For this review, take the finished solid that the model builds, in its own axes (mm). Face numbers are marked on the shaded views. A direction names the side the tool comes from. Give positions to 0.01 mm unless a question says otherwise; leave off trailing zeros. Order: outer loops, then holes, each group sorted by start corner. A loop starts at its lowest first (then second) coordinate and runs counter-clockwise, first axis right, second up. Notation, with made-up numbers: (83.25, 82) -> (104.25, 82) arc R27 cw to (104.25, 102) -> close; hole circle Ø7 at (11.25, 39.5). An arc over 180 degrees is marked (long way). Return JSON: item names as keys, results as strings. Group by question number.
1) Add section D-D (x = 80). Give the boundary of the cut face in (y, z), then the cut area to 3 significant figures.
2) For the marked faces 5 and 6, list the 3-axis set-ups (+Z, -Z, +X, -X, +Y, -Y) from which the entire face can be reached by the end or side of a thin tool; tool diameter is ignored.
3) Add section C-C (z = 15.75). Give the boundary of the cut face in (x, y), then the cut area to 3 significant figures.
4) Add section A-A (y = 16). Give the boundary of the cut face in (x, z), then the cut area to 4 significant figures.
5) To check wall thickness, follow line 1 along X through (y, z) = (40.5, 10); line 2 along X through (y, z) = (-32.5, 13.5); line 3 along X through (y, z) = (34, 10.5). State the ranges of each line that lie inside material, in increasing order.
6) Insertion check: P1, Ø8.5, axis at x = 80, z = 10, coming from the +Y side. The pin has a flat end and moves straight along its axis. Give the tip position at first contact, or say it passes through.
7) The part is to be moulded in two halves that separate along X. For the marked faces 1, 2, 3 and 4, say which applies: released by +X, released by -X, zero draft, split by the parting line, or undercut.
8) Add section B-B (x = 17). Give the boundary of the cut face in (y, z), then the cut area to 3 significant figures.
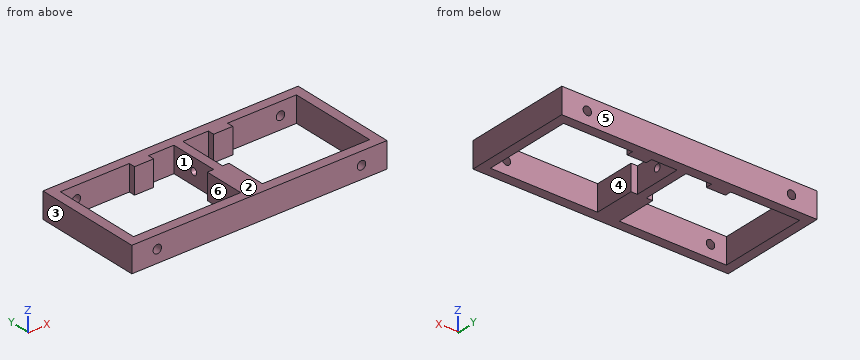
Autodesk Fusion 360 part; units mm, degrees
sketch "Sketch1" plane through (0, 0, 0) normal (0, 0, 1) x (1, 0, 0)
  line L0 (80, 0) -> (-80, 0) construction
  line L1 (100, 42.5) -> (-100, 42.5)
  line L2 (-100, 42.5) -> (-100, -42.5)
  line L3 (-100, -42.5) -> (100, -42.5)
  line L4 (100, -42.5) -> (100, 42.5)
  circle A0 centre (80, 0) radius 2.75
  circle A1 centre (-80, 0) radius 2.75
  line L5 (-90, 35) -> (-3.5, 35)
  line L6 (3.5, 35) -> (90, 35)
  line L7 (3.5, -35) -> (90, -35)
  line L8 (-3.5, -35) -> (-90, -35)
  line L9 (-3.5, 35) -> (-3.5, -3)
  line L10 (3.5, -3) -> (3.5, 35)
  line L11 (3.5, -3) -> (8.5, -3)
  line L12 (-3.5, -3) -> (-8.5, -3)
  line L13 (8.5, -3) -> (8.5, -35)
  line L14 (-8.5, -3) -> (-8.5, -35)
  line L15 (-90, 35) -> (-92.5, 35)
  line L16 (-92.5, 35) -> (-92.5, -35)
  line L17 (-92.5, -35) -> (-90, -35)
  line L18 (90, 35) -> (92.5, 35)
  line L19 (92.5, 35) -> (92.5, -35)
  line L20 (92.5, -35) -> (90, -35)
  line L21 (-23.5, 35) -> (-23.5, 30)
  line L22 (-23.5, 30) -> (-38.5, 30)
  line L23 (-38.5, 30) -> (-38.5, 35)
  line L24 (23.5, 35) -> (23.5, 30)
  line L25 (23.5, 30) -> (38.5, 30)
  line L26 (38.5, 30) -> (38.5, 35)
  dimension "d9" = 160
  dimension "d12" = 200
  dimension "d13" = 85
  dimension "d14" = 5.5
  dimension "d15" = 5.5
  dimension "d46" = 7
  dimension "d47" = 38
  dimension "d55" = 5
  dimension "d56" = 5
  dimension "d66" = 2.5
  dimension "d67" = 2.5
  dimension "d68" = 20
  dimension "d69" = 15
  dimension "d70" = 20
  dimension "d71" = 15
sketch "Sketch3" plane through (0, -42.5, 0) normal (0, -1, 0) x (1, 0, 0)
  line L0 (-100, 0) -> (100, 0)
  line L1 (100, 0) -> (100, 20)
  line L2 (100, 20) -> (-100, 20)
  line L3 (-100, 20) -> (-100, 0)
  line L4 (-100, 10) -> (-80, 10) construction
  line L5 (100, 10) -> (80, 10) construction
  dimension "d50" = 20
  dimension "d51" = 20
sketch "Sketch4" plane through (-3.5, 0, 0) normal (-1, 0, 0) x (0, -1, 0)
  line L0 (-35, 0) -> (3, 0)
  line L1 (3, 0) -> (3, 20)
  line L2 (3, 20) -> (-35, 20)
  line L3 (-35, 20) -> (-35, 0)
  line L4 (-35, 10) -> (3, 10) construction
  line L5 (-16, 20) -> (-16, 0) construction
  circle A0 centre (-16, 10) radius 2.75
  dimension "d62" = 5.5
extrude "Extrude7" add sketch "Sketch1" along normal blind 20 contours L1 L2 L3 L4 | L5 L21 L22 L23 | L6 L24 L25 L26
hole "Hole6" at (-80, -42.5, 10) at (80, -42.5, 10) direction (0, 1, 0) diameter 6.6 depth 85 tip angle 180
hole "Hole7" at (-3.5, 16, 10) direction (1, 0, 0) diameter 5.5 depth 7 tip angle 180
Evaluation:
{
 "1": {"outline": "(-42.5, 0) -> (-35, 0) -> (-35, 6.7) -> (-42.5, 6.7) -> close; (-42.5, 13.3) -> (-35, 13.3) -> (-35, 20) -> (-42.5, 20) -> close; (35, 0) -> (42.5, 0) -> (42.5, 6.7) -> (35, 6.7) -> close; (35, 13.3) -> (42.5, 13.3) -> (42.5, 20) -> (35, 20) -> close", "area": "201 mm^2"},
 "2": {"face 5": "+Z, -Z, +X, -X, +Y", "face 6": "+Z, -Z"},
 "3": {"outline": "(-100, -42.5) -> (100, -42.5) -> (100, 42.5) -> (-100, 42.5) -> close; hole (-92.5, -35) -> (-8.5, -35) -> (-8.5, -3) -> (-3.5, -3) -> (-3.5, 35) -> (-23.5, 35) -> (-23.5, 30) -> (-38.5, 30) -> (-38.5, 35) -> (-92.5, 35) -> close; hole (3.5, -3) -> (8.5, -3) -> (8.5, -35) -> (92.5, -35) -> (92.5, 35) -> (38.5, 35) -> (38.5, 30) -> (23.5, 30) -> (23.5, 35) -> (3.5, 35) -> close", "area": "5,010 mm^2"},
 "4": {"outline": "(-100, 0) -> (-92.5, 0) -> (-92.5, 20) -> (-100, 20) -> close; (-3.5, 0) -> (3.5, 0) -> (3.5, 7.25) -> (-3.5, 7.25) -> close; (-3.5, 12.75) -> (3.5, 12.75) -> (3.5, 20) -> (-3.5, 20) -> close; (92.5, 0) -> (100, 0) -> (100, 20) -> (92.5, 20) -> close", "area": "401.5 mm^2"},
 "5": {"line 1": "-100 to -83.3, -76.7 to 76.7, 83.3 to 100", "line 2": "-100 to -92.5, -8.5 to 8.5, 92.5 to 100", "line 3": "-100 to -92.5, -38.5 to -23.5, -3.5 to 3.5, 23.5 to 38.5, 92.5 to 100"},
 "6": {"P1": "y = 42.5"},
 "7": {"face 1": "undercut", "face 2": "zero draft", "face 3": "released by -X", "face 4": "undercut"},
 "8": {"outline": "(-42.5, 0) -> (-35, 0) -> (-35, 20) -> (-42.5, 20) -> close; (35, 0) -> (42.5, 0) -> (42.5, 20) -> (35, 20) -> close", "area": "300 mm^2"}
}
